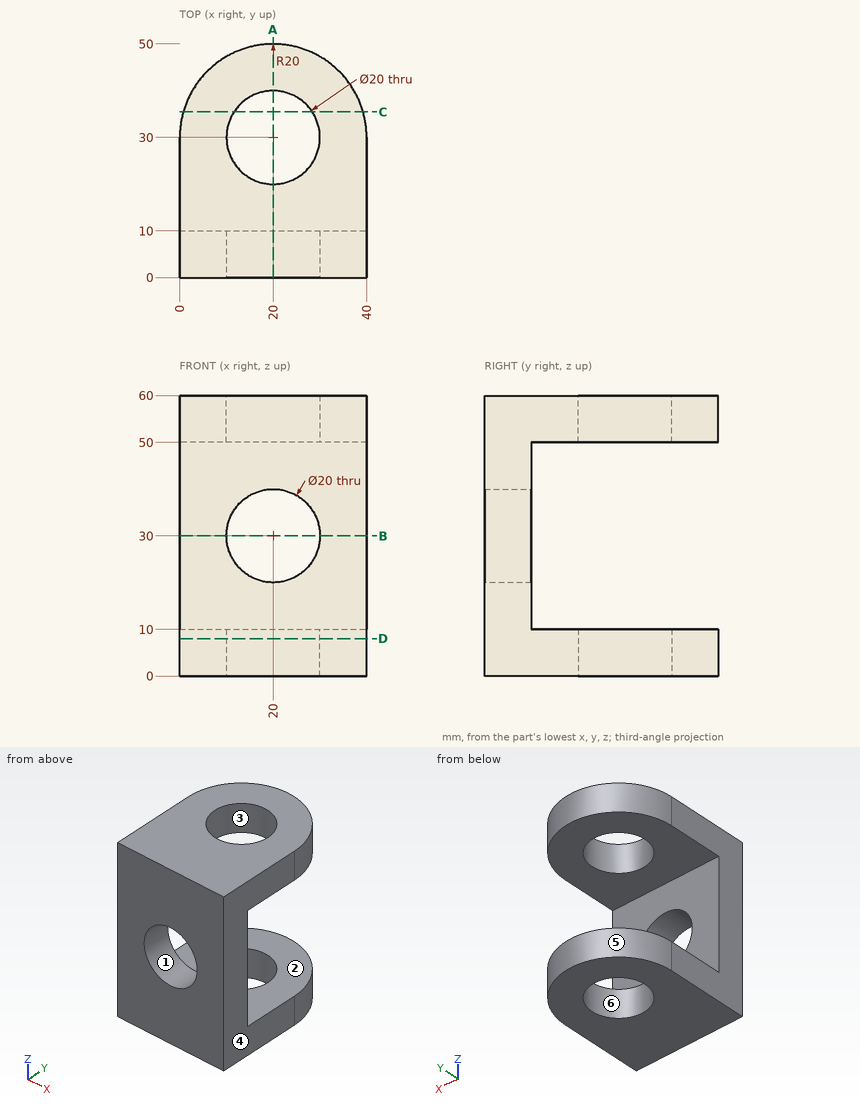
Job drawing, mm, ordinate dimensions from the low corner. One solid piece. A direction names the side the tool comes from. Round coordinates to 2 decimals unless told otherwise and drop trailing zeros. Loops run counter-clockwise (first coordinate to the right, second up) from the corner with the lowest first, then second, coordinate; pieces in that order, holes last. Notation, with made-up numbers: (12, 51) -> (41, 51) arc R15 cw to (41, 62) -> close; hole circle Ø9 at (-2, -0.75). An arc over 180 degrees is marked (long way). Use CSV: the item, a comma, the result in double quotes. Start each with the question number.
Q1. Saw through at A-A on x = 20. Give the cut face in (y, z).
Q2. Drill centre lines: L1, parallel to X at y = 4.25, z = 30; L2, parallel to Y at x = 20, z = 7; L3, parallel to Z at x = 5, y = 22. Where is each one in solid material? Low to high.
Q3. Saw through at D-D on z = 8. Give the cut face in (x, y).
Q4. Saw through at C-C on y = 35.5. Give the cut face in (x, z), and give its area (3 significant figures).
Q5. Mould opens along Y. For the marked faces 3, 4, 5 and 6 say: +Y half, -Y half, draft (parallel to the pull), parting line (faces both ways), or undercut.
Q6. Flat gauge pin, fed straight in: pin 1 Ø5 at (x, z) = (26.5, 25) entering from +Y. Where does the tip first touch, or does it go through?
Q7. Saw through at B-B on z = 30. Give the cut face in (x, y), and give its area (3 significant figures).
Q8. Which spindle directions (+Z, -Z, +X, -X, +Y, -Y) get a long thin tool onto all of the face, cutting with end or side? Do the marked faces 1 and 2. Say none if no direction does.
Solutions:
1,outline,"(0, 0) -> (20, 0) -> (20, 10) -> (10, 10) -> (10, 20) -> (0, 20) -> close; (0, 40) -> (10, 40) -> (10, 50) -> (20, 50) -> (20, 60) -> (0, 60) -> close; (40, 0) -> (50, 0) -> (50, 10) -> (40, 10) -> close; (40, 50) -> (50, 50) -> (50, 60) -> (40, 60) -> close"
2,L1,"x = 0 to 10, 30 to 40"
2,L2,"y = 0 to 20, 40 to 50"
2,L3,"z = 0 to 10, 50 to 60"
3,outline,"(0, 0) -> (40, 0) -> (40, 30) arc R20 ccw to (0, 30) -> close; hole circle Ø20 at (20, 30)"
4,outline,"(0.77, 0) -> (11.65, 0) -> (11.65, 10) -> (0.77, 10) -> close; (0.77, 50) -> (11.65, 50) -> (11.65, 60) -> (0.77, 60) -> close; (28.35, 0) -> (39.23, 0) -> (39.23, 10) -> (28.35, 10) -> close; (28.35, 50) -> (39.23, 50) -> (39.23, 60) -> (28.35, 60) -> close"
4,area,"435 mm^2"
5,face 3,"undercut"
5,face 4,"draft"
5,face 5,"+Y half"
5,face 6,"undercut"
6,pin 1,"stops at y = 10"
7,outline,"(0, 0) -> (10, 0) -> (10, 10) -> (0, 10) -> close; (30, 0) -> (40, 0) -> (40, 10) -> (30, 10) -> close"
7,area,"200 mm^2"
8,face 1,"+Y, -Y"
8,face 2,"+X, -X, +Y"
